Could you check a few things on this model? Use its own coordinates, in mm. A direction names the side the tool comes from. Give positions to 0.01 mm unless a question says otherwise; leave off trailing zeros. Loops run counter-clockwise (first coordinate to the right, second up) from the corner with the lowest first, then second, coordinate; pieces in that order, holes last. Notation, with made-up numbers: M 3.25,57 L 8.25,57 A16 ccw 8.25,74 Z; hole C -18.75,46 d6. An arc over 180 degrees is marked long. Return JSON: item names as keys, results as strings. Group by question number.
1. For faces 4 (the flat face through (-7.8, 4.93, -49.92)), 5 (the flat face through (-2.4, 10, -42.3)), 6 (the flat face through (4, 20, -29)), which set-ups out of +Z, -Z, +X, -X, +Y, -Y let a thin tool reach every point of the face, with its end or its side?
2. For pin 1 (5 mm diameter, centred on x = -1.5, z = -39, fed in from -Y); pin 2 (3 mm diameter, centred on x = 8, z = -51.5, fed in from +Y); pin 3 (8 mm diameter, centred on y = 26.5, z = -48, fed in from +X), each with a flat end and sliding along its axis, tell me the tip position at first contact or that it passes through.
3. Please list where these lines run through material, in increasing order: line 1 (X direction, y = 6.5, z = -40); line 2 (X direction, y = 22, z = -40); line 3 (Z direction, x = 0, y = 4).
4. If we section it at C-C (y = 30): Write out the boundary of the cut face in (x, z), plus the area to 3 significant figures.
5. If we section it at D-D (y = 17): Write out the boundary of the cut face in (x, z).
6. If we mould it in two halves opening along X, with no side actions, what happens to faces 1 (the flat face through (0, 35, -36)), 2 (the cylindrical face through (-5.99, 4.93, -46.03)), 3 (the flat face through (19, 5, -40))? For each: +X half, -X half, draft (parallel to the pull), parting line (faces both ways), or undercut.
7. If we section it at A-A (z = -40): Write out the boundary of the cut face in (x, y), plus the area to 3 significant figures.
8. If we section it at B-B (x = 0): Write out the boundary of the cut face in (y, z).
```python
from build123d import *
from build123d.topology import SkipClean

# Parameters (mm, degrees)
SKETCH_1_R          = 5
SKETCH_1_R_2        = 1.5
EXTRUDE_2_DEPTH     = 3
CUT_EXTRUDE_START   = -37
SKETCH_2_R          = 1.5
CUT_EXTRUDE_1_DEPTH = 37
SKETCH_3_W          = 38
SKETCH_3_H          = 6.73766493
EXTRUDE_3_DEPTH     = 3
SKETCH_5_W          = 53.60328953
SKETCH_5_H          = 19.816992683
CUT_EXTRUDE_2_DEPTH = 3
SKETCH_6_W          = 38
SKETCH_6_H          = 40
EXTRUDE_5_DEPTH     = 7
SKETCH_8_W          = 38
SKETCH_8_H          = 8
CUT_EXTRUDE_4_DEPTH = 44
SKETCH_9_R          = 5
CUT_EXTRUDE_5_DEPTH = 44
CUT_EXTRUDE_6_DEPTH = 44
SKETCH_13_R         = 8.5
EXTRUDE_6_DEPTH     = 25
SKETCH_14_R         = 3
CUT_EXTRUDE_7_DEPTH = 25
EXTRUDE_7_DEPTH     = 4
FILLET_1_R          = 10


with BuildPart() as part:
    # Sketch 1 → Extrude 2 (new body)
    with BuildSketch(Plane(origin=(0, 0, 0), x_dir=(1, 0, 0), z_dir=(0, 1, 0))):
        with BuildLine():
            Line((0, 0), (19, 0))
            Line((19, 0), (19, 64))
            ThreePointArc((19, 64), (0, 66.760766922), (-19, 64))
            Line((-19, 64), (-19, 0))
            Line((-19, 0), (0, 0))
        make_face()
        with Locations(Location((0, 40, 0), (0, 0, 270))):
            Circle(SKETCH_1_R, mode=Mode.SUBTRACT)
        with Locations(Location((-16.171572875, 2.828427125, 0), (0, 0, 270))):
            Circle(SKETCH_1_R_2, mode=Mode.SUBTRACT)
        with Locations(Location((-16.171572875, 61.171572875, 0), (0, 0, 270))):
            Circle(SKETCH_1_R_2, mode=Mode.SUBTRACT)
        with Locations(Location((16.171572875, 61.171572875, 0), (0, 0, 90))):
            Circle(SKETCH_1_R_2, mode=Mode.SUBTRACT)
        with Locations(Location((16.171572875, 2.828427125, 0), (0, 0, 90))):
            Circle(SKETCH_1_R_2, mode=Mode.SUBTRACT)
        with BuildLine():
            Line((10.606601718, 19.929208429), (10.606601718, 16.885025549))
            ThreePointArc((10.606601718, 16.885025549), (0, 16), (-10.606601718, 16.885025549))
            Line((-10.606601718, 16.885025549), (-10.606601718, 19.929208429))
            ThreePointArc((-10.606601718, 19.929208429), (0, 19), (10.606601718, 19.929208429))
        make_face(mode=Mode.SUBTRACT)
        with BuildLine():
            Line((-8.131727984, 46.01040764), (-11.66726189, 49.545941546))
            ThreePointArc((-11.66726189, 49.545941546), (-11.66726189, 51.66726189), (-9.545941546, 51.66726189))
            Line((-9.545941546, 51.66726189), (-6.01040764, 48.131727984))
            ThreePointArc((-6.01040764, 48.131727984), (-6.01040764, 46.01040764), (-8.131727984, 46.01040764))
        make_face(mode=Mode.SUBTRACT)
        with BuildLine():
            Line((6.01040764, 48.131727984), (9.545941546, 51.66726189))
            ThreePointArc((9.545941546, 51.66726189), (11.66726189, 51.66726189), (11.66726189, 49.545941546))
            Line((11.66726189, 49.545941546), (8.131727984, 46.01040764))
            ThreePointArc((8.131727984, 46.01040764), (6.01040764, 46.01040764), (6.01040764, 48.131727984))
        make_face(mode=Mode.SUBTRACT)
        with BuildLine():
            Line((8.131727984, 33.98959236), (11.66726189, 30.454058454))
            ThreePointArc((11.66726189, 30.454058454), (11.66726189, 28.33273811), (9.545941546, 28.33273811))
            Line((9.545941546, 28.33273811), (6.01040764, 31.868272016))
            ThreePointArc((6.01040764, 31.868272016), (6.01040764, 33.98959236), (8.131727984, 33.98959236))
        make_face(mode=Mode.SUBTRACT)
        with BuildLine():
            Line((-6.01040764, 31.868272016), (-9.545941546, 28.33273811))
            ThreePointArc((-9.545941546, 28.33273811), (-11.66726189, 28.33273811), (-11.66726189, 30.454058454))
            Line((-11.66726189, 30.454058454), (-8.131727984, 33.98959236))
            ThreePointArc((-8.131727984, 33.98959236), (-6.01040764, 33.98959236), (-6.01040764, 31.868272016))
        make_face(mode=Mode.SUBTRACT)
        with BuildLine():
            Line((-10.606601718, 60.070791571), (-10.606601718, 63.114974451))
            ThreePointArc((-10.606601718, 63.114974451), (0, 64), (10.606601718, 63.114974451))
            Line((10.606601718, 63.114974451), (10.606601718, 60.070791571))
            ThreePointArc((10.606601718, 60.070791571), (0, 61), (-10.606601718, 60.070791571))
        make_face(mode=Mode.SUBTRACT)
    extrude(amount=EXTRUDE_2_DEPTH)

    # Sketch 2 → Cut-Extrude 1 (cut)
    with BuildSketch(Plane(origin=(0, 3, 0), x_dir=(1, 0, 0), z_dir=(0, 1, 0)).offset(CUT_EXTRUDE_START)):
        Polygon((0, 24), (-19, 24), (-19, 0), (19, 0), (19, 24), align=None)
        with Locations((-16.171572875, 2.828427125)):
            Circle(SKETCH_2_R, mode=Mode.SUBTRACT)
        with Locations((16.171572875, 2.828427125)):
            Circle(SKETCH_2_R, mode=Mode.SUBTRACT)
        with BuildLine():
            Line((-10.606601718, 16.885025549), (-10.606601718, 19.929208429))
            ThreePointArc((-10.606601718, 19.929208429), (0, 19), (10.606601718, 19.929208429))
            Line((10.606601718, 19.929208429), (10.606601718, 16.885025549))
            ThreePointArc((10.606601718, 16.885025549), (0, 16), (-10.606601718, 16.885025549))
        make_face(mode=Mode.SUBTRACT)
    extrude(amount=CUT_EXTRUDE_1_DEPTH, mode=Mode.SUBTRACT)

    # Sketch 3 → Extrude 3 (add)
    with BuildSketch(Plane.XZ):
        with Locations((0, -60.631167535)):
            Rectangle(SKETCH_3_W, SKETCH_3_H)
    extrude(amount=-EXTRUDE_3_DEPTH)

    # Sketch 5 → Cut-Extrude 2 (cut)
    with BuildSketch(Plane(origin=(0, 3, 0), x_dir=(1, 0, 0), z_dir=(0, 1, 0))):
        with Locations((7.801644765, 73.908496342)):
            Rectangle(SKETCH_5_W, SKETCH_5_H)
    extrude(amount=-CUT_EXTRUDE_2_DEPTH, mode=Mode.SUBTRACT)

    # Sketch 6 → Extrude 5 (add)
    with BuildSketch(Plane(origin=(0, 3, 0), x_dir=(1, 0, 0), z_dir=(0, 1, 0))):
        with Locations((0, 44)):
            Rectangle(SKETCH_6_W, SKETCH_6_H)
    extrude(amount=EXTRUDE_5_DEPTH)

    # Sketch 8 → Cut-Extrude 4 (cut)
    with BuildSketch(Plane(origin=(0, 0, 0), x_dir=(-1, 0, 0), z_dir=(0, -1, 0))):
        with Locations((0, 60)):
            Rectangle(SKETCH_8_W, SKETCH_8_H)
    extrude(amount=-CUT_EXTRUDE_4_DEPTH, mode=Mode.SUBTRACT)

    # Sketch 9 → Cut-Extrude 5 (cut)
    with BuildSketch(Plane.XZ):
        with Locations(Location((0, -40, 0), (0, 0, 90))):
            Circle(SKETCH_9_R)
    extrude(amount=-CUT_EXTRUDE_5_DEPTH, mode=Mode.SUBTRACT)

    # Sketch 11 → Cut-Extrude 6 (cut)
    with BuildSketch(Plane.XZ):
        with BuildLine():
            Line((11.66726189, -30.454058454), (8.131727984, -33.98959236))
            ThreePointArc((8.131727984, -33.98959236), (6.01040764, -33.98959236), (6.01040764, -31.868272016))
            Line((6.01040764, -31.868272016), (9.545941546, -28.33273811))
            ThreePointArc((9.545941546, -28.33273811), (11.66726189, -28.33273811), (11.66726189, -30.454058454))
        make_face()
        with BuildLine():
            Line((9.545941546, -51.66726189), (6.01040764, -48.131727984))
            ThreePointArc((6.01040764, -48.131727984), (6.01040764, -46.01040764), (8.131727984, -46.01040764))
            Line((8.131727984, -46.01040764), (11.66726189, -49.545941546))
            ThreePointArc((11.66726189, -49.545941546), (11.66726189, -51.66726189), (9.545941546, -51.66726189))
        make_face()
        with BuildLine():
            Line((-11.66726189, -49.545941546), (-8.131727984, -46.01040764))
            ThreePointArc((-8.131727984, -46.01040764), (-6.01040764, -46.01040764), (-6.01040764, -48.131727984))
            Line((-6.01040764, -48.131727984), (-9.545941546, -51.66726189))
            ThreePointArc((-9.545941546, -51.66726189), (-11.66726189, -51.66726189), (-11.66726189, -49.545941546))
        make_face()
        with BuildLine():
            Line((-9.545941546, -28.33273811), (-6.01040764, -31.868272016))
            ThreePointArc((-6.01040764, -31.868272016), (-6.01040764, -33.98959236), (-8.131727984, -33.98959236))
            Line((-8.131727984, -33.98959236), (-11.66726189, -30.454058454))
            ThreePointArc((-11.66726189, -30.454058454), (-11.66726189, -28.33273811), (-9.545941546, -28.33273811))
        make_face()
    extrude(amount=-CUT_EXTRUDE_6_DEPTH, mode=Mode.SUBTRACT)

    # Sketch 13 → Extrude 6 (add)
    with SkipClean():  # the faces are left unmerged after this step: merging them gives an invalid solid
        with BuildSketch(Plane(origin=(0, 10, 0), x_dir=(1, 0, 0), z_dir=(0, 1, 0))):
            with Locations(Location((0, 40, 0), (0, 0, 134.99989234))):
                Circle(SKETCH_13_R)
        extrude(amount=EXTRUDE_6_DEPTH)
    add(part.part.scale(1), mode=Mode.REPLACE)  # the faces are merged on a copy

    # Sketch 14 → Cut-Extrude 7 (cut)
    with BuildSketch(Plane(origin=(0, 35, 0), x_dir=(1, 0, 0), z_dir=(0, 1, 0))):
        with Locations(Location((0, 40, 0), (0, 0, 270))):
            Circle(SKETCH_14_R)
    extrude(amount=-CUT_EXTRUDE_7_DEPTH, mode=Mode.SUBTRACT)

    # Sketch 15 → Extrude 7 (add, symmetric)
    with BuildSketch(Plane(origin=(0, 0, 0), x_dir=(0, 0, -1), z_dir=(1, 0, 0))):
        Polygon((31.5, 35), (24, 10), (31.5, 10), (32.928568569, 10), (32.928568569, 35), align=None)
    extrude(amount=EXTRUDE_7_DEPTH, both=True)

    # Fillet 1
    fillet_1_edges = [part.edges().sort_by_distance(p)[0] for p in [
        (-19, 5, -24),
        (19, 5, -24),
        (19, 5, -56),
        (-19, 5, -56),
    ]]
    fillet(fillet_1_edges, radius=FILLET_1_R)


solid = part.part
```
Answer:
{
 "1": {"face 4": "+Y, -Y", "face 5": "-Y", "face 6": "+Z, +X, +Y"},
 "2": {"pin 1": "stops at y = 10", "pin 2": "stops at y = 10", "pin 3": "stops at x = 7.5"},
 "3": {"line 1": "x = -19 to -5, 5 to 19", "line 2": "x = -8.5 to -3, 3 to 8.5", "line 3": "z = -56 to -45, -35 to -24"},
 "4": {"outline": "M -4,-32.5 A8.5 ccw long 4,-32.5 L 4,-30 L -4,-30 Z; hole C 0,-40 d6", "area": "213 mm²"},
 "5": {"outline": "M -4,-32.5 A8.5 ccw long 4,-32.5 L 4,-26.1 L -4,-26.1 Z; hole C 0,-40 d6"},
 "6": {"face 1": "draft", "face 2": "undercut", "face 3": "+X half"},
 "7": {"outline": "M -19,0 L -5,0 L -5,10 L -3,10 L -3,35 L -8.5,35 L -8.5,10 L -19,10 Z; M 3,10 L 5,10 L 5,0 L 19,0 L 19,10 L 8.5,10 L 8.5,35 L 3,35 Z", "area": "555 mm²"},
 "8": {"outline": "M 0,-56 L 10,-56 L 10,-48.5 L 35,-48.5 L 35,-43 L 10,-43 L 10,-45 L 0,-45 Z; M 0,-35 L 10,-35 L 10,-37 L 35,-37 L 35,-31.5 L 10,-24 L 0,-24 Z"}
}
